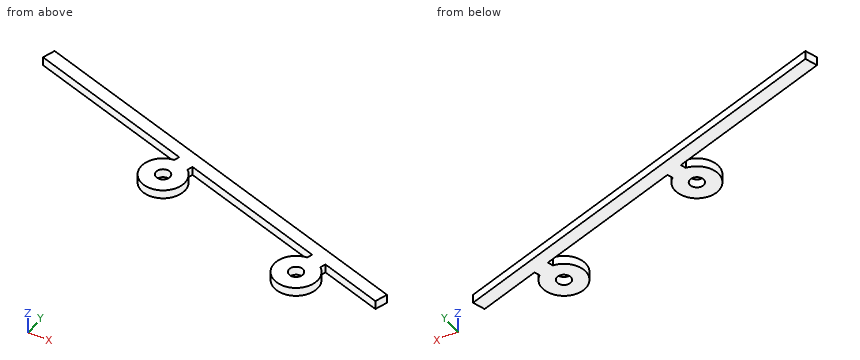
Autodesk Inventor part; units mm, degrees
ref_plane "YZ Plane" through (0, 0, 0) normal (1, 0, 0) x (0, 1, 0)
ref_plane "XZ Plane" through (0, 0, 0) normal (0, 1, 0) x (-1, 0, 0)
ref_plane "XY Plane" through (0, 0, 0) normal (0, 0, 1) x (1, 0, 0)
ref_plane "Work Plane1" through (0, 0, 0) normal (0, 0, 1) x (1, 0, 0)
sketch "Sketch1" plane through (0, 0, 0) normal (0, 0, 1) x (1, 0, 0)
  circle A0 centre (0, 28) radius 1.6
  arc A1 (3.5119, -2.971) -> (3.88, 2.471) centre (0, 0) ccw
  arc A2 (4.2226, 26.7696) -> (3.88, 2.471) centre (48.0455, 14) ccw
  arc A3 (4.2226, 26.7696) -> (-4.2226, 26.7696) centre (0, 28) ccw
  arc A4 (-3.88, 2.471) -> (-4.2226, 26.7696) centre (-48.0455, 14) ccw
  arc A5 (-3.88, 2.471) -> (-3.5119, -2.971) centre (0, 0) ccw
  arc A6 (-3.9828, -12.5413) -> (-3.5119, -2.971) centre (-19.1125, -7) ccw
  arc A7 (-3.9828, -12.5413) -> (3.9828, -12.5413) centre (0, -14) ccw
  arc A8 (3.5119, -2.971) -> (3.9828, -12.5413) centre (19.1125, -7) ccw
  circle A9 centre (0, 0) radius 1.6
  circle A10 centre (0, 21) radius 1.6
  circle A11 centre (0, 28) radius 1.6
  circle A12 centre (0, 14) radius 1.6
  circle A13 centre (0, 7) radius 1.6
  circle A14 centre (0, -7) radius 1.6
  circle A15 centre (0, -14) radius 1.6
  circle A16 centre (0, 28) radius 5
  line L0 (18, 28.1562) -> (18.9553, 31)
  line L1 (18.9553, 31) -> (-75.839, 62.8438)
  line L2 (-75.839, 62.8438) -> (-76.7944, 60)
  line L3 (-76.7944, 60) -> (18, 28.1562)
  line L4 (3.7683, 32.937) -> (-0.0235, 34.2107)
  line L5 (-0.0235, 34.2107) -> (-0.4366, 32.9809)
  line L6 (-0.4366, 32.9809) -> (3.3552, 31.7071)
  line L7 (3.3552, 31.7071) -> (3.7683, 32.937)
  line L8 (9.4559, 31.0263) -> (9.0428, 29.7965)
  circle A17 centre (9.4794, 24.8156) radius 5
  line L9 (9.0428, 29.7965) -> (12.8346, 28.5228)
  line L10 (12.8346, 28.5228) -> (13.2477, 29.7526)
  line L11 (-9.5029, 37.3951) -> (-9.9161, 36.1653)
  circle A18 centre (-9.4794, 31.1844) radius 5
  line L12 (-9.9161, 36.1653) -> (-6.1243, 34.8915)
  line L13 (-6.1243, 34.8915) -> (-5.7112, 36.1213)
  line L14 (-0.0235, 34.2107) -> (-0.4366, 32.9809)
  circle A19 centre (0, 28) radius 5
  line L15 (-0.4366, 32.9809) -> (3.3552, 31.7071)
  line L16 (3.3552, 31.7071) -> (3.7683, 32.937)
  line L17 (-18.9824, 40.5795) -> (-19.3955, 39.3497)
  circle A20 centre (-18.9589, 34.3688) radius 5
  line L18 (-19.3955, 39.3497) -> (-15.6037, 38.0759)
  line L19 (-15.6037, 38.0759) -> (-15.1906, 39.3057)
  line L20 (-9.5029, 37.3951) -> (-9.9161, 36.1653)
  circle A21 centre (-9.4794, 31.1844) radius 5
  line L21 (-9.9161, 36.1653) -> (-6.1243, 34.8915)
  line L22 (-6.1243, 34.8915) -> (-5.7112, 36.1213)
  line L23 (-28.4618, 43.7639) -> (-28.8749, 42.534)
  circle A22 centre (-28.4383, 37.5531) radius 5
  line L24 (-28.8749, 42.534) -> (-25.0832, 41.2603)
  line L25 (-25.0832, 41.2603) -> (-24.67, 42.4901)
  line L26 (-18.9824, 40.5795) -> (-19.3955, 39.3497)
  circle A23 centre (-18.9589, 34.3688) radius 5
  line L27 (-19.3955, 39.3497) -> (-15.6037, 38.0759)
  line L28 (-15.6037, 38.0759) -> (-15.1906, 39.3057)
  line L29 (-37.9412, 46.9483) -> (-38.3544, 45.7184)
  circle A24 centre (-37.9177, 40.7375) radius 5
  line L30 (-38.3544, 45.7184) -> (-34.5626, 44.4447)
  line L31 (-34.5626, 44.4447) -> (-34.1495, 45.6745)
  line L32 (-28.4618, 43.7639) -> (-28.8749, 42.534)
  circle A25 centre (-28.4383, 37.5531) radius 5
  line L33 (-28.8749, 42.534) -> (-25.0832, 41.2603)
  line L34 (-25.0832, 41.2603) -> (-24.67, 42.4901)
  line L35 (-47.4207, 50.1326) -> (-47.8338, 48.9028)
  circle A26 centre (-47.3972, 43.9219) radius 5
  line L36 (-47.8338, 48.9028) -> (-44.042, 47.6291)
  line L37 (-44.042, 47.6291) -> (-43.6289, 48.8589)
  line L38 (-37.9412, 46.9483) -> (-38.3544, 45.7184)
  circle A27 centre (-37.9177, 40.7375) radius 5
  line L39 (-38.3544, 45.7184) -> (-34.5626, 44.4447)
  line L40 (-34.5626, 44.4447) -> (-34.1495, 45.6745)
  line L41 (-56.9001, 53.317) -> (-57.3132, 52.0872)
  circle A28 centre (-56.8766, 47.1063) radius 5
  line L42 (-57.3132, 52.0872) -> (-53.5215, 50.8134)
  line L43 (-53.5215, 50.8134) -> (-53.1083, 52.0433)
  line L44 (-47.4207, 50.1326) -> (-47.8338, 48.9028)
  circle A29 centre (-47.3972, 43.9219) radius 5
  line L45 (-47.8338, 48.9028) -> (-44.042, 47.6291)
  line L46 (-44.042, 47.6291) -> (-43.6289, 48.8589)
  line L47 (-66.3795, 56.5014) -> (-66.7927, 55.2716)
  circle A30 centre (-66.3561, 50.2907) radius 5
  line L48 (-66.7927, 55.2716) -> (-63.0009, 53.9978)
  line L49 (-63.0009, 53.9978) -> (-62.5878, 55.2276)
  line L50 (-56.9001, 53.317) -> (-57.3132, 52.0872)
  circle A31 centre (-56.8766, 47.1063) radius 5
  line L51 (-57.3132, 52.0872) -> (-53.5215, 50.8134)
  line L52 (-53.5215, 50.8134) -> (-53.1083, 52.0433)
  line L53 (-75.859, 59.6858) -> (-76.2721, 58.456)
  circle A32 centre (-75.8355, 53.4751) radius 5
  line L54 (-76.2721, 58.456) -> (-72.4803, 57.1822)
  line L55 (-72.4803, 57.1822) -> (-72.0672, 58.412)
  line L56 (-66.3795, 56.5014) -> (-66.7927, 55.2716)
  circle A33 centre (-66.3561, 50.2907) radius 5
  line L57 (-66.7927, 55.2716) -> (-63.0009, 53.9978)
  line L58 (-63.0009, 53.9978) -> (-62.5878, 55.2276)
  circle A34 centre (0, 28) radius 1.6
  circle A35 centre (-9.4794, 31.1844) radius 1.6
  circle A36 centre (-18.9589, 34.3688) radius 1.6
  circle A37 centre (-28.4383, 37.5531) radius 1.6
  circle A38 centre (-37.9177, 40.7375) radius 1.6
  circle A39 centre (-47.3972, 43.9219) radius 1.6
  circle A40 centre (-56.8766, 47.1063) radius 1.6
  circle A41 centre (-66.3561, 50.2907) radius 1.6
  circle A42 centre (-75.8355, 53.4751) radius 1.6
  circle A43 centre (9.4794, 24.8156) radius 1.6
  circle A44 centre (0, 28) radius 1.6
  circle A45 centre (-9.4794, 31.1844) radius 1.6
  circle A46 centre (-18.9589, 34.3688) radius 1.6
  circle A47 centre (-28.4383, 37.5531) radius 1.6
  circle A48 centre (-37.9177, 40.7375) radius 1.6
  circle A49 centre (-47.3972, 43.9219) radius 1.6
  circle A50 centre (-56.8766, 47.1063) radius 1.6
  circle A51 centre (-66.3561, 50.2907) radius 1.6
  dimension "d0" = 10
  dimension "d1" = 18
  dimension "d2" = 3
  dimension "d3" = 3
  dimension "d4" = 100
  dimension "d5" = 32
  dimension "d6" = 4
  dimension "d11" = 10
  dimension "d14" = 10
  dimension "d19" = 10
  dimension "d22" = 10
extrude "Extrusion1" add sketch "Sketch1" along normal blind 2 contours A16 A4 A3 A2 | A2 A3 A4 A16 L6 | L5 L3 L7 A16 | A16 L6 | L3 L2 L1 L0 | A24 L30 | L29 L3 L31 A24 | A24 L30
properties part number "leaf-lid"
Could you check a few things on this model? Use its own coordinates, in mm. Round coordinates to 2 decimals unless told otherwise and drop trailing zeros. Order: outer loops, then holes, each group sorted by start corner. A loop starts at its lowest first (then second) coordinate and runs counter-clockwise, first axis right, second up.
Q1. Imagine slicing it at D-D, the plane x = -6. List the corners of the cut face in (y, z) for me.
Geometry says:
outline: (36.22, 0) - (39.38, 0) - (39.38, 2) - (36.22, 2) - close
Q2. I'm going to push a flat-ended pin straight in: P1, Ø3, axis at x = 0, y = 28, coming from the -Z side. Where does the tip first touch, or does it pass through?
Geometry says:
P1: passes through
Q3. Please list where these lines run through material, in increasing order: probe 1 along Y at (x, z) = (-46, 1.75); probe 2 along Y at (x, z) = (-2, 1.2); probe 3 along Y at (x, z) = (-42.5, 1.35).
Geometry says:
probe 1: y = 49.66 to 52.82
probe 2: y = 23.42 to 32.58, 34.87 to 38.04
probe 3: y = 38.74 to 42.74, 48.48 to 51.64
Q4. Imagine slicing it at A-A, the plane y = 38. List the corners of the cut face in (x, z) for me.
Geometry says:
outline: (-42.1, 0) - (-33.73, 0) - (-33.73, 2) - (-42.1, 2) - close; (-11.3, 0) - (-1.88, 0) - (-1.88, 2) - (-11.3, 2) - close
Q5. Imagine slicing it at B-B, the plane z = 1.45. List the corners of the cut face in (x, y) for me.
Geometry says:
outline: (-76.79, 60) - (-37.94, 46.95) - (-38.35, 45.72) arc R5 ccw (long way) to (-34.56, 44.44) - (-34.15, 45.67) - (-0.02, 34.21) - (-0.44, 32.98) arc R5 ccw (long way) to (3.36, 31.71) - (3.77, 32.94) - (18, 28.16) - (18.96, 31) - (-75.84, 62.84) - close; hole circle Ø3.2 at (-37.92, 40.74); hole circle Ø3.2 at (0, 28)
Q6. Imagine slicing it at C-C, the plane x = -30. List the corners of the cut face in (y, z) for me, then the cut area to 3 significant figures.
Geometry says:
outline: (44.28, 0) - (47.45, 0) - (47.45, 2) - (44.28, 2) - close
area: 6.33 mm2
